```python
from build123d import *

# Parameters (mm, degrees)
EXTRUDE_1_DEPTH             = 5
SKETCH_46_W                 = 130
SKETCH_46_H                 = 20
CUT_EXTRUDE_31_DEPTH        = 5
SKETCH_8_R                  = 2.6
CUT_EXTRUDE_6_DEPTH         = 6
PATTERN_CIRCULAR_1_COUNT    = 3
CHAMFER_1_SIZE              = 5
CUT_EXTRUDE_4_DEPTH         = 6
SKETCH_9_R                  = 1.65
CUT_EXTRUDE_7_DEPTH         = 6
FILLET_1_R                  = 15
M4X0_7_4_D                  = 3.3
CUT_EXTRUDE_35_REACH        = 7
SKETCH_53_R                 = 2.1
CUT_EXTRUDE_37_DEPTH        = 5
PATTERN_LINEAR_1_COUNT      = 2
PATTERN_LINEAR_1_PITCH      = 20
PATTERN_LINEAR_1_COUNT_DIR2 = 2
PATTERN_LINEAR_1_PITCH_DIR2 = 20
CUT_EXTRUDE_38_REACH        = 7
SKETCH_54_R                 = 8.05
SKETCH_56_R                 = 1.6
CUT_EXTRUDE_40_DEPTH        = 10
SKETCH_55_W                 = 30
SKETCH_55_H                 = 40
CUT_EXTRUDE_39_DEPTH        = 10
FILLET_2_R                  = 1
M3X0_5_1_D                  = 2.5
M3X0_5_1_DEPTH              = 8.5
M3X0_5_1_TIP                = 0.751075774
M4X0_7_5_AT_2_COUNT         = 2
M4X0_7_5_AT_2_PITCH         = 126.194294641
M4X0_7_5_AT_3_COUNT         = 2
M4X0_7_5_AT_3_PITCH         = 125.39936204
M4X0_7_5_AT_4_COUNT         = 2
M4X0_7_5_AT_4_PITCH         = 54.083269132
M3X0_5_2_D                  = 2.5
M3X0_5_2_DEPTH              = 8.5
M3X0_5_2_TIP                = 0.751075774


with BuildPart() as part:
    # Sketch 1 → Extrude 1 (new body)
    with BuildSketch(Plane(origin=(0, 0, 0), x_dir=(1, 0, 0), z_dir=(0, 1, 0))):
        Polygon((85, 147.224318643), (-85, 147.224318643), (-170, 0), (-85, -147.224318643), (85, -147.224318643), (170, 0), align=None)
    extrude(amount=EXTRUDE_1_DEPTH)

    # Sketch 46 → Cut-Extrude 31 (cut)
    with BuildSketch(Plane(origin=(0, 5, 0), x_dir=(1, 0, 0), z_dir=(0, 1, 0))):
        with Locations((0, -137.224318643)):
            Rectangle(SKETCH_46_W, SKETCH_46_H)
    cut_extrude_31 = extrude(amount=-CUT_EXTRUDE_31_DEPTH, mode=Mode.SUBTRACT)

    # Sketch 8 → Cut-Extrude 6 (cut, through all)
    with BuildSketch(Plane(origin=(0, 5, 0), x_dir=(1, 0, 0), z_dir=(0, 1, 0))):
        with Locations((-27.5, -119.224318643)):
            Circle(SKETCH_8_R)
        with Locations((27.5, -119.224318643)):
            Circle(SKETCH_8_R)
        with Locations((-27.5, -107.224318643)):
            Circle(SKETCH_8_R)
        with Locations((27.5, -107.224318643)):
            Circle(SKETCH_8_R)
    cut_extrude_6 = extrude(amount=-CUT_EXTRUDE_6_DEPTH, mode=Mode.SUBTRACT)

    # Pattern Circular 1: Cut-Extrude 31, Cut-Extrude 6 ×3 about axis
    pattern_circular_1_axis = Axis((0, 0, 0), (0, 1, 0))
    for i in range(1, PATTERN_CIRCULAR_1_COUNT):
        add(cut_extrude_31.rotate(pattern_circular_1_axis, i * 360 / PATTERN_CIRCULAR_1_COUNT), mode=Mode.SUBTRACT)
        add(cut_extrude_6.rotate(pattern_circular_1_axis, i * 360 / PATTERN_CIRCULAR_1_COUNT), mode=Mode.SUBTRACT)

    # Chamfer 1
    chamfer_1_edges = [part.edges().sort_by_distance(p)[0] for p in [
        (-65, 2.5, 147.224318643),
        (-65, 2.5, 127.224318643),
        (65, 2.5, 127.224318643),
        (65, 2.5, 147.224318643),
        (160, 2.5, -17.320508076),
        (142.679491924, 2.5, -7.320508076),
        (77.679491924, 2.5, -119.903810568),
        (95, 2.5, -129.903810568),
        (-95, 2.5, -129.903810568),
        (-77.679491924, 2.5, -119.903810568),
        (-142.679491924, 2.5, -7.320508076),
        (-160, 2.5, -17.320508076),
    ]]
    chamfer(chamfer_1_edges, length=CHAMFER_1_SIZE)

    # Sketch 5 → Cut-Extrude 4 (cut, through all)
    with BuildSketch(Plane(origin=(0, 5, 0), x_dir=(1, 0, 0), z_dir=(0, 1, 0))):
        Polygon((-152.5, -30.310889132), (-107, -109.119200877), (-42.048094716, -71.619200877), (-87.548094716, 7.189110868), align=None)
    cut_extrude_4 = extrude(amount=-CUT_EXTRUDE_4_DEPTH, mode=Mode.SUBTRACT)

    # Sketch 9 → Cut-Extrude 7 (cut, through all)
    with BuildSketch(Plane(origin=(0, 5, 0), x_dir=(1, 0, 0), z_dir=(0, 1, 0))):
        with Locations((-89.491669751, -113.444518424)):
            Circle(SKETCH_9_R)
        with Locations((-147.491669751, -12.985571585)):
            Circle(SKETCH_9_R)
    cut_extrude_7 = extrude(amount=-CUT_EXTRUDE_7_DEPTH, mode=Mode.SUBTRACT)

    # Mirror 1: Cut-Extrude 4, Cut-Extrude 7 across plane
    add(cut_extrude_4.mirror(Plane(origin=(0, 0, 0), x_dir=(0, 0, 1), z_dir=(1, 0, 0))), mode=Mode.SUBTRACT)
    add(cut_extrude_7.mirror(Plane(origin=(0, 0, 0), x_dir=(0, 0, 1), z_dir=(1, 0, 0))), mode=Mode.SUBTRACT)

    # Fillet 1
    fillet_1_edges = [part.edges().sort_by_distance(p)[0] for p in [
        (170, 2.5, 0),
        (85, 2.5, 147.224318643),
        (-85, 2.5, 147.224318643),
        (-170, 2.5, 0),
    ]]
    fillet(fillet_1_edges, radius=FILLET_1_R)

    # M4x0.7 _4 (through all)
    with Locations(Plane(origin=(0, 5, 0), x_dir=(1, 0, 0), z_dir=(0, 1, 0))):
        with Locations((-72.869891486, -2.234282891), (-57.869891486, -28.215045005), (-42.869891486, -54.195807118)):
            m4x0_7_4 = Hole(M4X0_7_4_D / 2)

    # Mirror 2: M4x0.7 _4 across plane
    add(m4x0_7_4.mirror(Plane(origin=(0, 0, 0), x_dir=(0, 0, 1), z_dir=(1, 0, 0))), mode=Mode.SUBTRACT)

    # Sketch 51 → Cut-Extrude 35 (cut, up to next)
    with BuildSketch(Plane(origin=(0, 5, 0), x_dir=(1, 0, 0), z_dir=(0, 1, 0)), mode=Mode.PRIVATE) as cut_extrude_35_sk1:
        Polygon((20, 34.641016151), (-20, 34.641016151), (-40, 0), (-20, -34.641016151), (20, -34.641016151), (40, 0), align=None)
    cut_extrude_35_tool1 = extrude(cut_extrude_35_sk1.sketch, amount=-CUT_EXTRUDE_35_REACH, mode=Mode.PRIVATE) & part.part
    add(cut_extrude_35_tool1.solids().sort_by_distance((0, 5, 0))[0], mode=Mode.SUBTRACT)

    # Sketch 53 → Cut-Extrude 37 (cut)
    with BuildSketch(Plane(origin=(0, 5, 0), x_dir=(1, 0, 0), z_dir=(0, 1, 0))):
        with Locations((20, 127.224318643)):
            Circle(SKETCH_53_R)
    cut_extrude_37 = extrude(amount=-CUT_EXTRUDE_37_DEPTH, mode=Mode.SUBTRACT)

    # Pattern Linear 1: Cut-Extrude 37 2 × 2
    with Locations(*[(i * PATTERN_LINEAR_1_PITCH, 0, j * PATTERN_LINEAR_1_PITCH_DIR2) for i in range(PATTERN_LINEAR_1_COUNT) for j in range(PATTERN_LINEAR_1_COUNT_DIR2) if (i, j) != (0, 0)]):
        add(cut_extrude_37, mode=Mode.SUBTRACT)

    # Sketch 54 → Cut-Extrude 38 (cut, up to next)
    with BuildSketch(Plane(origin=(0, 5, 0), x_dir=(1, 0, 0), z_dir=(0, 1, 0)), mode=Mode.PRIVATE) as cut_extrude_38_sk1:
        with Locations((71.5, 135.224318643)):
            Circle(SKETCH_54_R)
    cut_extrude_38_tool1 = extrude(cut_extrude_38_sk1.sketch, amount=-CUT_EXTRUDE_38_REACH, mode=Mode.PRIVATE) & part.part
    add(cut_extrude_38_tool1.solids().sort_by_distance((71.5, 5, -135.224319))[0], mode=Mode.SUBTRACT)

    # Sketch 56 → Cut-Extrude 40 (cut)
    with BuildSketch(Plane(origin=(0, 0, 0), x_dir=(-1, 0, 0), z_dir=(0, -1, 0))):
        with Locations((34.6, 122.224318643)):
            Circle(SKETCH_56_R)
        with Locations((44.4, 122.224318643)):
            Circle(SKETCH_56_R)
        with Locations((44.4, 73.824318643)):
            Circle(SKETCH_56_R)
        with Locations((34.6, 73.824318643)):
            Circle(SKETCH_56_R)
    extrude(amount=-CUT_EXTRUDE_40_DEPTH, mode=Mode.SUBTRACT)

    # Sketch 55 → Cut-Extrude 39 (cut)
    with BuildSketch(Plane(origin=(0, 5, 0), x_dir=(1, 0, 0), z_dir=(0, 1, 0))):
        with Locations((-39.5, 98.024318643)):
            Rectangle(SKETCH_55_W, SKETCH_55_H)
    extrude(amount=-CUT_EXTRUDE_39_DEPTH, mode=Mode.SUBTRACT)

    # Fillet 2
    fillet_2_edges = [part.edges().sort_by_distance(p)[0] for p in [
        (-24.5, 2.5, -78.024318643),
        (-54.5, 2.5, -78.024318643),
        (-54.5, 2.5, -118.024318643),
        (-24.5, 2.5, -118.024318643),
    ]]
    fillet(fillet_2_edges, radius=FILLET_2_R)

    # M3x0.5 _1
    with Locations(Plane(origin=(0, 5, 0), x_dir=(1, 0, 0), z_dir=(0, 1, 0))):
        with Locations((-60.5, 104.524318643), (-60.5, 84.524318643), (-18.5, 84.524318643), (-18.5, 104.524318643)):
            Hole(M3X0_5_1_D / 2, depth=M3X0_5_1_DEPTH)
            with Locations((0, 0, -(M3X0_5_1_DEPTH + M3X0_5_1_TIP / 2))):  # 118° drill point
                Cone(0, M3X0_5_1_D / 2, M3X0_5_1_TIP, mode=Mode.SUBTRACT)

    # Sketch 61 → M4x0.7 _5 (revolve, cut)
    with BuildSketch(Plane(origin=(-50, 5, 95), x_dir=(0, 0, 1), z_dir=(1, 0, 0))):
        Polygon((0, 0), (0, 12.491420021), (1.65, 11.5), (1.65, 0), align=None)
    m4x0_7_5 = revolve(axis=Axis((-50, 11.35, 95), (0, -1, 0)), mode=Mode.SUBTRACT)

    # M4x0.7 _5 at 2: M4x0.7 _5 ×2
    with Locations(*[Vector(-0.554700196, 0, -0.832050294) * (i * M4X0_7_5_AT_2_PITCH) for i in range(1, M4X0_7_5_AT_2_COUNT)]):
        add(m4x0_7_5, mode=Mode.SUBTRACT)

    # M4x0.7 _5 at 3: M4x0.7 _5 ×2
    with Locations(*[Vector(-0.079745222, 0, -0.996815279) * (i * M4X0_7_5_AT_3_PITCH) for i in range(1, M4X0_7_5_AT_3_COUNT)]):
        add(m4x0_7_5, mode=Mode.SUBTRACT)

    # M4x0.7 _5 at 4: M4x0.7 _5 ×2
    with Locations(*[Vector(0.554700196, 0, -0.832050294) * (i * M4X0_7_5_AT_4_PITCH) for i in range(1, M4X0_7_5_AT_4_COUNT)]):
        add(m4x0_7_5, mode=Mode.SUBTRACT)

    # Mirror 3: M4x0.7 _5 across plane
    add(m4x0_7_5.mirror(Plane(origin=(0, 0, 0), x_dir=(0, 0, 1), z_dir=(1, 0, 0))), mode=Mode.SUBTRACT)

    # Mirror 3 copy 1 sketch → Mirror 3 copy 1 (revolve, cut)
    with BuildSketch(Plane(origin=(120, 5, -10), x_dir=(0, 0, 1), z_dir=(-1, 0, 0))):
        Polygon((0, 0), (0, -12.491420021), (1.65, -11.5), (1.65, 0), align=None)
    revolve(axis=Axis((120, 11.35, -10), (0, 1, 0)), mode=Mode.SUBTRACT)

    # Mirror 3 copy 2 sketch → Mirror 3 copy 2 (revolve, cut)
    with BuildSketch(Plane(origin=(60, 5, -30), x_dir=(0, 0, 1), z_dir=(-1, 0, 0))):
        Polygon((0, 0), (0, -12.491420021), (1.65, -11.5), (1.65, 0), align=None)
    revolve(axis=Axis((60, 11.35, -30), (0, 1, 0)), mode=Mode.SUBTRACT)

    # Mirror 3 copy 3 sketch → Mirror 3 copy 3 (revolve, cut)
    with BuildSketch(Plane(origin=(20, 5, 50), x_dir=(0, 0, 1), z_dir=(-1, 0, 0))):
        Polygon((0, 0), (0, -12.491420021), (1.65, -11.5), (1.65, 0), align=None)
    revolve(axis=Axis((20, 11.35, 50), (0, 1, 0)), mode=Mode.SUBTRACT)

    # M3x0.5 _2
    with Locations(Plane(origin=(0, 5, 0), x_dir=(1, 0, 0), z_dir=(0, 1, 0))):
        with Locations((-20, -77.224318643), (-20, -117.224318643), (20, -117.224318643), (20, -77.224318643)):
            Hole(M3X0_5_2_D / 2, depth=M3X0_5_2_DEPTH)
            with Locations((0, 0, -(M3X0_5_2_DEPTH + M3X0_5_2_TIP / 2))):  # 118° drill point
                Cone(0, M3X0_5_2_D / 2, M3X0_5_2_TIP, mode=Mode.SUBTRACT)


solid = part.part
```
Source: CAD feature listing. Evaluate the final solid. Frame: model axes, mm. A direction names the side the tool comes from. Give positions to 0.01 mm unless a question says otherwise; leave off trailing zeros. Loops run counter-clockwise (first coordinate to the right, second up) from the corner with the lowest first, then second, coordinate; pieces in that order, holes last. Notation, with made-up numbers: (-35, 33) - (19, 33) arc R22 cw to (19, 67) - close; hole circle Ø7 at (3, 61). An arc over 180 degrees is marked (long way). Use CSV: the item, a comma, the result in double quotes. Start each with the question number.
1. Section A-A (z = -93). Output: boundary loops of the cut face in (x, y).
2. Reachability of faces 1 (the flat face through (-74.979, 2.535, 90.632)), 2 (the flat face through (-88.697, 2.465, -140.82)), 3 (the flat face through (119.57, 2.54, 11.3)) from +Z, -Z, +X, -X, +Y, -Y: full face, straight path, thin tool, end or side. Return the list, or none.
3. Section B-B (y = 3.55). Count the separate pieces of the cut face and the enclosed holes in it, then the cut area to 3 significant figures.
4. Draft query along X for faces 4 (the flat face through (-119.57, 2.54, 11.3)), 5 (the flat face through (-2, 5, -35)), 6 (the cylindrical face through (-83.74, 2.54, 145.27)), 7 (the flat face through (74.979, 2.535, 90.632)). Return one class per face: +X half, -X half, draft (parallel to the pull), parting line (faces both ways), or undercut.
5. Pin query (flat end, axial travel): pin 1 (6 mm diameter, centred on x = 27.5, z = 119.22, fed in from -Y); pin 2 (1.5 mm diameter, centred on y = 4.5, z = 78, fed in from -X); pin 3 (1 mm diameter, centred on y = 2, z = -2.5, fed in from -X); pin 4 (2 mm diameter, centred on x = -125.5, y = 4.5, fed in from +Z). Return the tip coordinate at first contact, or that it passes through.
6. Ray query, L1, parallel to Z at x = 57, y = 2.3; L2, parallel to Z at x = -82.5, y = 1.05; L3, parallel to X at y = 3.35, z = -77.5. Return the intervals inside material, ascending.
Response:
1,outline,"(-93.21, 0) - (-54.5, 0) - (-54.5, 5) - (-93.21, 5) - close; (-24.5, 0) - (93.21, 0) - (93.21, 5) - (-24.5, 5) - close"
2,face 1,"-X, +Y, -Y"
2,face 2,"-Z, -X, +Y, -Y"
2,face 3,"+Y, -Y"
3,separate pieces,"1"
3,enclosed holes,"49"
3,area,"47,500 mm²"
4,face 4,"undercut"
4,face 5,"draft"
4,face 6,"-X half"
4,face 7,"+X half"
5,pin 1,"y = 0"
5,pin 2,"x = -54.4"
5,pin 3,"x = -167.55"
5,pin 4,"z = 15.3"
6,L1,"-147.22 to 26.81, 29.62 to 45.72, 80.25 to 127.22"
6,L2,"-147.22 to -122.69, -111.55 to 1.55, 94.97 to 145.9"
6,L3,"-102.16 to -81.71, -76.51 to 76.51, 81.71 to 102.16"
